```python
from build123d import *

# Parameters (mm, degrees)
F0_W           = 12
F0_H           = 12.475
F3_D           = 6
F4_D           = 3.3
F4_CBORE_D     = 6.5
F4_CBORE_DEPTH = 5
F5_R           = 0.5


with BuildPart() as f1:
    # F0 (on Right) → F1 (revolve)
    with BuildSketch(Plane.YZ):
        with Locations((0, 16.2625)):
            Rectangle(F0_W, F0_H)
    revolve(axis=Axis((0, 1.880541, 0), (0, 1, 0)))

    # F3 (through all)
    with Locations(Plane(origin=(0, 6, 0), x_dir=(-1, 0, 0), z_dir=(0, 1, 0))):
        with Locations((-13.081475, 13.081475), (13.081475, 13.081475), (-13.081475, -13.081475), (13.081475, -13.081475)):
            Hole(F3_D / 2)

    # F4 (through all)
    with Locations(Plane(origin=(0, 6, 0), x_dir=(-1, 0, 0), z_dir=(0, 1, 0))):
        with Locations((-18.5, 0), (0, -18.5), (18.5, 0), (0, 18.5)):
            CounterBoreHole(F4_D / 2, F4_CBORE_D / 2, F4_CBORE_DEPTH)

    # F5
    f5_edges = [f1.edges().sort_by_distance(p)[0] for p in [
        (0, 6, -22.5),
        (0, -6, -22.5),
        (0, 6, -10.025),
        (0, -6, -10.025),
        (0, 0, 10.025),
    ]]
    fillet(f5_edges, radius=F5_R)


solid = f1.part
```
Source: CAD feature listing. Evaluate the final solid. Frame: model axes, mm. A direction names the side the tool comes from. Round coordinates to 2 decimals unless told otherwise and drop trailing zeros. Put each result on its own line as item: value.
(1) First-contact query: pin 1 (5.5 mm diameter, centred on x = 0, z = 18.5, fed in from +Y); pin 2 (5 mm diameter, centred on x = 13.08, z = -13.08, fed in from -Y); pin 3 (3 mm diameter, centred on y = -1.5, z = 12, fed in from -X). Flat tips, straight axial feed; report the tip coordinate or a pass-through.
Solutions:
pin 1: y = 1
pin 2: through
pin 3: x = -19.9
(2) Pull-direction query (X, two-part tool) for faces 3 (the face through (-19.961, 0.077, 10.382)), 4 (the face through (5.2, -6, -9.5)), 5 (the face through (1, 1, 20)); classes: released by +X, released by -X, zero draft, split by the parting line, or undercut.
Solutions:
face 3: split by the parting line
face 4: zero draft
face 5: undercut
(3) Access query for faces 1 (the face through (0.423, 3.535, 21.722)), 2 (the face through (15.943, -0.084, -12.18)). Directions: +Z, -Z, +X, -X, +Y, -Y. A direction counts if a zero-diameter tool reaches every point of the face in a straight line with its end or side. Return the directions, or none.
Solutions:
face 1: +Y
face 2: +Y, -Y
(4) Ray query, line 1 (Z direction, x = -15, y = 0); line 2 (X direction, y = -4.25, z = -14); line 3 (X direction, y = -4, z = -13). Return the intervals inside material, ascending. Write a range as [from, to].
Solutions:
line 1: [-16.77, -15.39], [-10.78, 10.78], [15.39, 16.77]
line 2: [-17.61, -15.94], [-10.23, 10.23], [15.94, 17.61]
line 3: [-18.36, -16.08], [-10.08, 10.08], [16.08, 18.36]
(5) Section A-A, the plane z = 0. State how many separate pieces and enclosed holes the cut face has, and give its area (3 significant figures).
Solutions:
separate pieces: 4
enclosed holes: 0
area: 188 mm²
